Input: part model. Units: mm. Frame: model coordinates. A direction names the side the tool comes from. Give positions to 0.01 mm unless a question says otherwise; leave off trailing zeros. Loops run counter-clockwise (first coordinate to the right, second up) from the corner with the lowest first, then second, coordinate; pieces in that order, holes last.
from build123d import *

# Parameters (mm, degrees)
SKETCH5_R               = 0.9
CUT_EXTRUDE2_DEPTH      = 6.5
CUT_EXTRUDE2_DEPTH_BACK = 6.5


with BuildPart() as part:
    # Sketch3 → Revolve19 (revolve)
    with BuildSketch(Plane.XY):
        Polygon((262.558388758, -144.573704322), (262.558388758, -144.073704322), (272.558388758, -144.073704322), (272.558388758, -143.073704322), (261.558388758, -143.073704322), (261.558388758, -144.323704322), (261.558388758, -148.073704322), (263.058388758, -148.073704322), (263.058388758, -144.573704322), align=None)
    revolve(axis=Axis((263.058388758, -148.573704322, 0), (1, 0, 0)))

    # Sketch5 → Cut-Extrude2 (cut, two sides)
    with BuildSketch(Plane.XY) as cut_extrude2_sk:
        with Locations((269.808388758, -148.573704322)):
            Circle(SKETCH5_R)
    extrude(amount=CUT_EXTRUDE2_DEPTH, mode=Mode.SUBTRACT)
    extrude(cut_extrude2_sk.sketch, amount=-CUT_EXTRUDE2_DEPTH_BACK, mode=Mode.SUBTRACT)


solid = part.part
(1) Cut plane A-A (y = -148.75). Return the cut outline in (x, z).
Values follow:
outline: (261.56, -5.5) - (268.93, -5.5) - (268.93, -4.5) - (262.56, -4.5) - (262.56, -4) - (263.06, -4) - (263.06, -0.47) - (261.56, -0.47) - close; (261.56, 0.47) - (263.06, 0.47) - (263.06, 4) - (262.56, 4) - (262.56, 4.5) - (268.93, 4.5) - (268.93, 5.5) - (261.56, 5.5) - close; (270.69, -5.5) - (272.56, -5.5) - (272.56, -4.5) - (270.69, -4.5) - close; (270.69, 4.5) - (272.56, 4.5) - (272.56, 5.5) - (270.69, 5.5) - close
(2) Cut plane B-B (z = 0). Return the cut outline in (x, y).
Values follow:
outline: (261.56, -154.07) - (272.56, -154.07) - (272.56, -153.07) - (262.56, -153.07) - (262.56, -152.57) - (263.06, -152.57) - (263.06, -149.07) - (261.56, -149.07) - close; (261.56, -148.07) - (263.06, -148.07) - (263.06, -144.57) - (262.56, -144.57) - (262.56, -144.07) - (272.56, -144.07) - (272.56, -143.07) - (261.56, -143.07) - close
(3) Mould query, pull axis Y, two halves, no side actions, for faces 1 (the cylindrical face through (266.98, -146.04, -4.88)), 2 (the cylindrical face through (262.8, -144.76, 1.2)), 3 (the flat face through (272.558, -144, 1)). Classes: +Y half, -Y half, draft (parallel to the pull), parting line (faces both ways), or undercut.
Values follow:
face 1: parting line
face 2: undercut
face 3: draft
(4) Ray query, probe 1 along Z at (x, y) = (263, -146.25); probe 2 along X at (y, z) = (-151, 2); probe 3 along Y at (x, z) = (269, 3). Return the intervals inside material, ascending.
Values follow:
probe 1: z = -4.99 to -3.85, -3.26 to 3.26, 3.85 to 4.99
probe 2: x = 261.56 to 263.06
probe 3: y = -153.18 to -151.93, -145.22 to -143.96
(5) Cut plane D-D (y = -150). Return the cut outline in (x, z).
Values follow:
outline: (261.56, -5.31) - (272.56, -5.31) - (272.56, -4.27) - (262.56, -4.27) - (262.56, -3.74) - (263.06, -3.74) - (263.06, 3.74) - (262.56, 3.74) - (262.56, 4.27) - (272.56, 4.27) - (272.56, 5.31) - (261.56, 5.31) - close
(6) Pin query (flat end, axial travel): pin 1 Ø1.5 at (x, z) = (270, 1.5) entering from +Y; pin 2 Ø2.5 at (y, z) = (-150.5, 1) entering from +X. Return the tip coordinate at first contact, or that it passes through.
Values follow:
pin 1: stops at y = -143.13
pin 2: stops at x = 263.06
(7) Reachability of faces 4 (the cylindrical face through (270.292, -147.815, -4.947)), 5 (the cylindrical face through (267.628, -146.497, -3.992)) from +Z, -Z, +X, -X, +Y, -Y: full face, straight path, thin tool, end or side. Return the list, or none.
Values follow:
face 4: +Z, -Z
face 5: +X
(8) Cut plane C-C (x = 264.5). Return the cut outline in (y, z), and give its area (3 significant figures).
Values follow:
outline: circle Ø11 at (-148.57, 0); hole circle Ø9 at (-148.57, 0)
area: 31.4 mm2
